Source: CAD feature listing. Evaluate the final solid. Frame: model axes, mm. A direction names the side the tool comes from. Give positions to 0.01 mm unless a question says otherwise; leave off trailing zeros. Loops run counter-clockwise (first coordinate to the right, second up) from the corner with the lowest first, then second, coordinate; pieces in that order, holes last. Notation, with made-up numbers: M -25.75,21 L 6.25,21 A10 cw 6.25,26 Z; hole C 53.5,-23.5 d4. An arc over 180 degrees is marked long. Answer in a Markdown table with one row per item.
```python
from build123d import *

# Parameters (mm, degrees)
F1_DEPTH = 39.878
F2_R     = 13.9954
F3_DEPTH = 39.879
F4_DEPTH = 39.879
F5_DEPTH = 39.879
F6_R     = 2.5019
F7_DEPTH = 11.938


with BuildPart() as f1:
    # F0 (on Top) → F1 (new body)
    with BuildSketch(Plane.XY):
        Polygon((-25.9969, -19.939), (25.9969, -19.939), (25.9969, 7.9502), (14.0081, 19.939), (-14.0081, 19.939), (-25.9969, 7.9502), align=None)
        Polygon((14.0081, 19.939), (25.9969, 7.9502), (25.9969, 19.939), align=None)
        Polygon((-25.9969, 19.939), (-25.9969, 7.9502), (-14.0081, 19.939), align=None)
    extrude(amount=F1_DEPTH)

    # F2 (on face) → F3 (cut, through all)
    with BuildSketch(Plane.XY.offset(39.878)):
        Circle(F2_R)
    extrude(amount=-F3_DEPTH, mode=Mode.SUBTRACT)

    # F0 (on Top) → F4 (cut, through all)
    with BuildSketch(Plane.XY):
        Polygon((14.0081, 19.939), (25.9969, 7.9502), (25.9969, 19.939), align=None)
    extrude(amount=F4_DEPTH, mode=Mode.SUBTRACT)

    # F0 (on Top) → F5 (cut, through all)
    with BuildSketch(Plane.XY):
        Polygon((-25.9969, 19.939), (-25.9969, 7.9502), (-14.0081, 19.939), align=None)
    extrude(amount=F5_DEPTH, mode=Mode.SUBTRACT)

    # F6 (on face) → F7 (cut)
    with BuildSketch(Plane.XZ.offset(19.939)):
        with Locations((17.9959, 31.877)):
            Circle(F6_R)
        with Locations((17.9959, 8.001)):
            Circle(F6_R)
        with Locations((-17.9959, 8.001)):
            Circle(F6_R)
        with Locations((-17.9959, 31.877)):
            Circle(F6_R)
    extrude(amount=-F7_DEPTH, mode=Mode.SUBTRACT)


solid = f1.part
```
Q1. Reachability of faces 4 (the flat face through (-25.997, -6, 20)), 5 (the cylindrical face through (-16.84, -14.05, 29.66)) from +Z, -Z, +X, -X, +Y, -Y: full face, straight path, thin tool, end or side. Return the list, or none.
Values follow:
| item | result |
|---|---|
| face 4 | +Z, -Z, -X, +Y, -Y |
| face 5 | -Y |
Q2. Section query D-D (y = 0). Output: boundary loops of the cut face in (x, z).
Values follow:
| item | result |
|---|---|
| outline | M -26,0 L -14,0 L -14,39.88 L -26,39.88 Z; M 14,0 L 26,0 L 26,39.88 L 14,39.88 Z |
Q3. Mould query, pull axis X, two halves, no side actions, for faces 1 (the flat face through (0, 19.939, 20)), 2 (the flat face through (25.997, -6, 20)), 3 (the cylindrical face through (6.458, -12.416, 20.218)). Classes: +X half, -X half, draft (parallel to the pull), parting line (faces both ways), or undercut.
Values follow:
| item | result |
|---|---|
| face 1 | draft |
| face 2 | +X half |
| face 3 | undercut |
Q4. Section query A-A (x = 0). Output: boundary loops of the cut face in (y, z), plus the area to 3 significant figures.
Values follow:
| item | result |
|---|---|
| outline | M -19.94,0 L -14,0 L -14,39.88 L -19.94,39.88 Z; M 14,0 L 19.94,0 L 19.94,39.88 L 14,39.88 Z |
| area | 474 mm^2 |
Q5. Ray query, probe 1 along Y at (x, z) = (0, 13); probe 2 along Y at (x, z) = (-12.5, 28); probe 3 along X at (y, z) = (11.5, 7). Return the intervals inside material, ascending. Write a range as from..to.
Values follow:
| item | result |
|---|---|
| probe 1 | -19.94..-14, 14..19.94 |
| probe 2 | -19.94..-6.29, 6.29..19.94 |
| probe 3 | -22.45..-7.98, 7.98..22.45 |
Q6. Contact query for a flat-ended pin moving along its axis: pin 1 Ø1.5 at (x, z) = (-19, 9) entering from -Y. Output: stop coordinate, or through.
Values follow:
| item | result |
|---|---|
| pin 1 | y = -8 |
Q7. Section query B-B (y = -9.5). Output: boundary loops of the cut face in (x, z), plus the area to 3 significant figures.
Values follow:
| item | result |
|---|---|
| outline | M -26,0 L -10.28,0 L -10.28,39.88 L -26,39.88 Z; M 10.28,0 L 26,0 L 26,39.88 L 10.28,39.88 Z; hole C -18,8 d5; hole C -18,31.88 d5; hole C 18,8 d5; hole C 18,31.88 d5 |
| area | 1,180 mm^2 |
Q8. Section query C-C (z = 36.5). Output: boundary loops of the cut face in (x, y), plus the area to 3 significant figures.
Values follow:
| item | result |
|---|---|
| outline | M -26,-19.94 L 26,-19.94 L 26,7.95 L 14.01,19.94 L -14.01,19.94 L -26,7.95 Z; hole C 0,0 d27.99 |
| area | 1,310 mm^2 |
